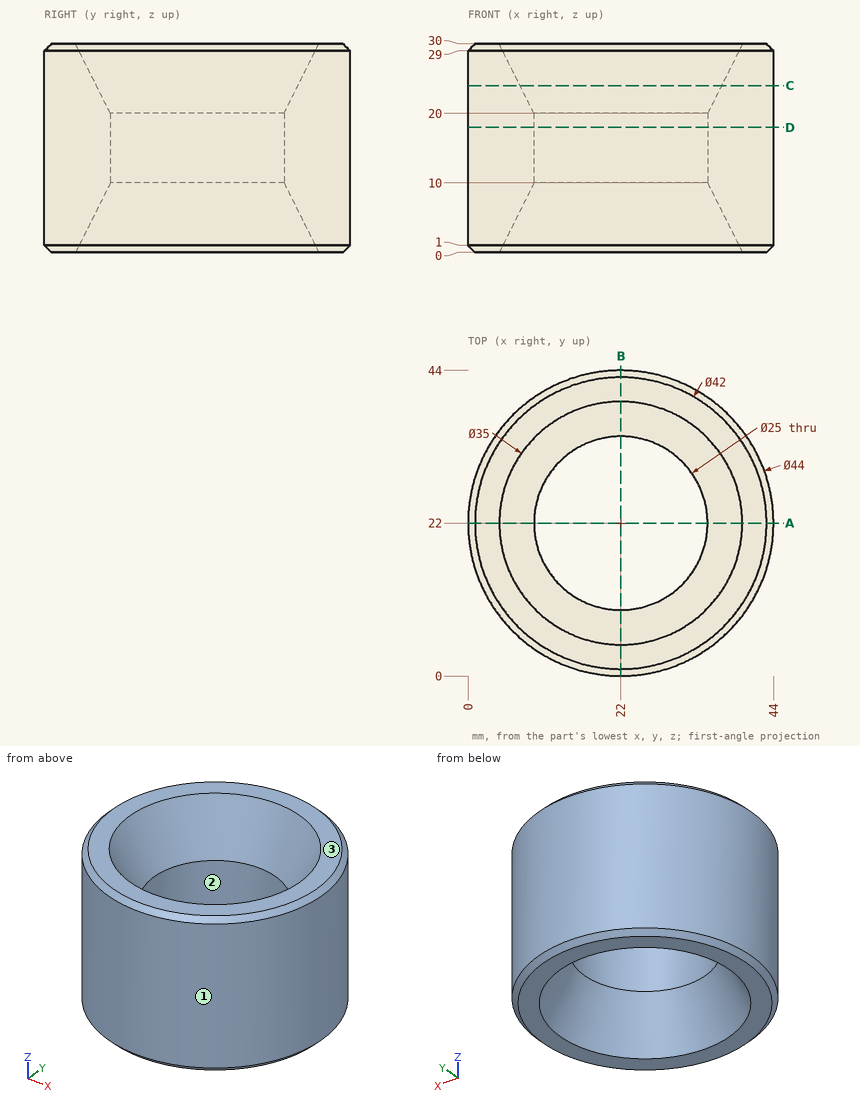
Could you check a few things on this drawing? It's one solid part, dimensions in mm from its lowest x, y, z. Round coordinates to 2 decimals unless told otherwise and drop trailing zeros. Order: outer loops, then holes, each group sorted by start corner. A loop starts at its lowest first (then second) coordinate and runs counter-clockwise, first axis right, second up. Notation, with made-up numbers: M 25.25,10 L 68.25,10 A28 ccw 68.25,44 Z; hole C 53.5,43.5 d1. An arc over 180 degrees is marked long. Return JSON: item names as keys, results as strings. Group by question number.
1. If we section it at C-C on z = 24: List the corners of the cut face in (x, y) for me.
2. Please list where these lines run through material, in increasing order: probe 1 along Y at (x, z) = (22, 14); probe 2 along Y at (x, z) = (15, 21); probe 3 along X at (y, z) = (30, 6.75).
3. If we section it at A-A on y = 22: List the corners of the cut face in (x, z) for me.
4. If we mould it in two halves opening along X, with no side actions, what happens to the marked faces 1, 2 and 3? For each: pulls with the +X half, pulls with the -X half, needs draft (parallel to the pull), parting line crosses it, or undercut.
5. If we section it at D-D on z = 18: List the corners of the cut face in (x, y) for me.
6. I'm going to push flat-ended pins straight in: pin 1 Ø8 at (x, z) = (5, 4.5) entering from -Y; pin 2 Ø8 at (x, z) = (20, 14) entering from -Y; pin 3 Ø1.5 at (x, z) = (37, 17.5) entering from -Y. Where does each tip first touch, or does it pass through?
Reply:
{
 "1": {"outline": "C 22,22 d44; hole C 22,22 d29"},
 "2": {"probe 1": "0 to 9.5, 34.5 to 44", "probe 2": "1.14 to 11.05, 32.95 to 42.86", "probe 3": "1.51 to 10.36, 33.64 to 42.49"},
 "3": {"outline": "M 0,1 L 1,0 L 4.5,0 L 9.5,10 L 9.5,20 L 4.5,30 L 1,30 L 0,29 Z; M 34.5,10 L 39.5,0 L 43,0 L 44,1 L 44,29 L 43,30 L 39.5,30 L 34.5,20 Z"},
 "4": {"face 1": "parting line crosses it", "face 2": "undercut", "face 3": "needs draft"},
 "5": {"outline": "C 22,22 d44; hole C 22,22 d25"},
 "6": {"pin 1": "y = 4.25", "pin 2": "y = 0", "pin 3": "y = 5.24"}
}
